Build history of the part. All positions in model axes, mm. A direction names the side the tool comes from. Round coordinates to 2 decimals unless told otherwise and drop trailing zeros. Write each loop counter-clockwise with the first axis right and the second up, starting at its lowest first coordinate (ties: lowest second). Pieces come first, ordered by that corner, then holes. Notation, with made-up numbers: M 22.25,36.5 L 76.25,36.5 A15 cw 76.25,42.5 Z; hole C 2.5,2.25 d9. An arc over 180 degrees is marked long. Write item = value, one per line.
from build123d import *

# Parameters (mm, degrees)
F1_DEPTH = 19.05
F2_R     = 0.508
F3_DEPTH = 12.7


with BuildPart() as f1:
    # F0 (on Front) → F1 (new body)
    with BuildSketch(Plane.XZ):
        Polygon((-9.511831, 0), (-22.211831, -21.997045), (3.188169, -21.997045), align=None)
    extrude(amount=F1_DEPTH)

    # F2 (on face) → F3 (cut)
    with BuildSketch(Plane.XZ.offset(19.05)):
        with Locations((-18.891316, -19.739211)):
            Circle(F2_R)
        with Locations((-14.926066, -19.739211)):
            Circle(F2_R)
        with Locations((-5.508598, -19.739211)):
            Circle(F2_R)
        with Locations((-0.693653, -19.739211)):
            Circle(F2_R)
        with Locations((-10.217332, -19.739211)):
            Circle(F2_R)
        with Locations((-12.199957, -15.419921)):
            Circle(F2_R)
        with Locations((-7.704876, -15.419921)):
            Circle(F2_R)
        with Locations((-3.455166, -15.455325)):
            Circle(F2_R)
        with Locations((-8.076196, -7.064574)):
            Circle(F2_R)
        with Locations((-13.828542, -11.242247)):
            Circle(F2_R)
        with Locations((-5.721022, -11.242247)):
            Circle(F2_R)
        with Locations((-9.544656, -3.417961)):
            Circle(F2_R)
        with Locations((-11.314857, -7.064574)):
            Circle(F2_R)
        with Locations((-9.662744, -11.242247)):
            Circle(F2_R)
        with Locations((-16.342226, -15.419921)):
            Circle(F2_R)
    extrude(amount=-F3_DEPTH, mode=Mode.SUBTRACT)


solid = f1.part
1. Flat gauge pins, fed straight in: pin 1 (0.6 mm diameter, centred on x = -5.72, z = -11.24, fed in from -Y); pin 2 (6 mm diameter, centred on y = -9, z = -13, fed in from -X); pin 3 (1.5 mm diameter, centred on x = -12, y = -16.5, fed in from +Z). Where does each tip first touch, or does it go through?
Responses:
pin_1 = -6.35
pin_2 = -18.75
pin_3 = -3.01
2. Tool access for faces 4 (the face through (-0.804, -12.789, -20.235)), 5 (the face through (-10, -9, -21.997)): list every direction of +Z, -Z, +X, -X, +Y, -Y with a clear straight run to the whole face (end or side of a thin tool).
Responses:
face_4 = -Y
face_5 = -Z, +X, -X, +Y, -Y
3. Band-saw the part on C-C (y = -5). List the corners of the cut face in (x, z), plus the area to 3 significant figures.
Responses:
outline = M -22.21,-22 L 3.19,-22 L -9.51,0 Z
area = 279 mm²
4. Band-saw the part on D-D (x = 1.25). List the corners of the cut face in (y, z).
Responses:
outline = M -19.05,-22 L 0,-22 L 0,-18.64 L -19.05,-18.64 Z
5. Band-saw the part on A-A (y = -12). Count the separate pieces of the cut face and the enclosed holes in it, plus the area to 3 significant figures.
Responses:
separate_pieces = 1
enclosed_holes = 15
area = 267 mm²
6. Mould opens along Z. For faces 1 (the face through (-3.073, -9.392, -11.153)), 2 (the face through (-10, -19.05, -16)), 3 (the face through (-10, -12.8, -20.2)) say: pulls with the +Z half, pulls with the -Z half, needs draft (parallel to the pull), parting line crosses it, or undercut.
Responses:
face_1 = pulls with the +Z half
face_2 = needs draft
face_3 = undercut
7. Probe probe 1 along Z at (x, y) = (-14, -7.5); probe 2 along Z at (x, y) = (-15, -14.75); probe 3 along X at (y, z) = (-8, -15.5). List the from-to ranges inside material, lowest first.
Responses:
probe_1 = -22 to -11.72, -10.76 to -7.77
probe_2 = -22 to -20.24, -19.24 to -9.51
probe_3 = -18.46 to -16.84, -15.84 to -12.7, -11.7 to -8.21, -7.2 to -3.96, -2.95 to -0.56
8. Band-saw the part on B-B (z = -12.25). List the corners of the cut face in (x, y), plus the area to 3 significant figures.
Responses:
outline = M -16.58,-19.05 L -2.44,-19.05 L -2.44,0 L -16.58,0 Z
area = 269 mm²
